Verification items for the finished model (mm, model axes). Coordinates: 2 decimals unless noted, no trailing zeros. Order: outer loops, then holes, each group sorted by start corner. A loop starts at its lowest first (then second) coordinate and runs counter-clockwise, first axis right, second up. Notation, with made-up numbers: (24, 35.25) - (31, 35.25) arc R6 ccw to (31, 41.25) - close; hole circle Ø10 at (60.25, 14). An arc over 180 degrees is marked (long way). One line per question, with ' | ' between items. Start each with the question number.
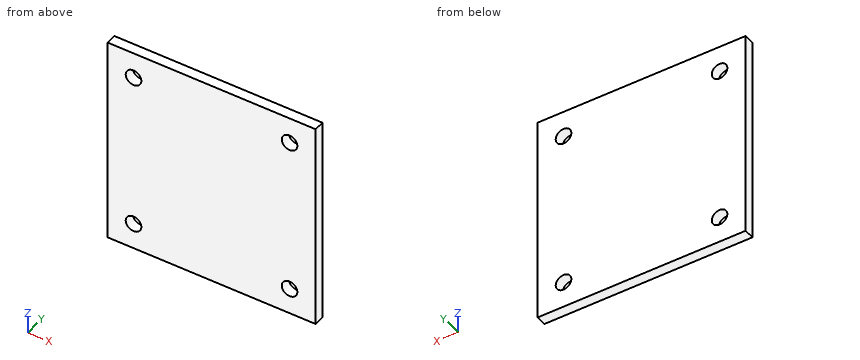
from build123d import *

# Parameters (mm, degrees)
SKETCH1_W           = 40
SKETCH1_H           = 40
BOSS_EXTRUDE1_DEPTH = 2
SKETCH2_R           = 1.5
CUT_EXTRUDE1_DEPTH  = 2


with BuildPart() as part:
    # Sketch1 → Boss-Extrude1 (new body)
    with BuildSketch(Plane(origin=(0, 0, 0), x_dir=(1, 0, 0), z_dir=(0, 1, 0))):
        with Locations((20, 20)):
            Rectangle(SKETCH1_W, SKETCH1_H)
    extrude(amount=BOSS_EXTRUDE1_DEPTH)

    # Sketch2 → Cut-Extrude1 (cut)
    with BuildSketch(Plane.XZ):
        with Locations((35, -5)):
            Circle(SKETCH2_R)
        with Locations((35, -35)):
            Circle(SKETCH2_R)
        with Locations((5, -5)):
            Circle(SKETCH2_R)
        with Locations((5, -35)):
            Circle(SKETCH2_R)
    extrude(amount=-CUT_EXTRUDE1_DEPTH, mode=Mode.SUBTRACT)


solid = part.part
Item 1: Section check C-C (x = 35). Record the cut outline in (y, z), then the cut area to 3 significant figures.
Item 2: Gauge pin test, flat end, axial feed: pin 1 (2.5 mm diameter, centred on x = 5, z = -35, fed in from -Y). Record the tip position at first contact, or that the pin passes through.
Item 3: Section check B-B (z = -5). Record the cut outline in (x, y), then the cut area to 3 significant figures.
Item 4: Section check A-A (y = 1.05). Record the cut outline in (x, z).
Item 5: Thickness scan on probe 1 along Z at (x, y) = (35, 0.6); probe 2 along Z at (x, y) = (4, 1.65); probe 3 along X at (y, z) = (0.35, -4.5). Record the ranges inside material, lowest first. Write a range as from..to.
Completed:
1) outline: (0, -40) - (2, -40) - (2, -36.5) - (0, -36.5) - close; (0, -33.5) - (2, -33.5) - (2, -6.5) - (0, -6.5) - close; (0, -3.5) - (2, -3.5) - (2, 0) - (0, 0) - close | area: 68.0 mm^2
2) pin 1: passes through
3) outline: (0, 0) - (3.5, 0) - (3.5, 2) - (0, 2) - close; (6.5, 0) - (33.5, 0) - (33.5, 2) - (6.5, 2) - close; (36.5, 0) - (40, 0) - (40, 2) - (36.5, 2) - close | area: 68.0 mm^2
4) outline: (0, -40) - (40, -40) - (40, 0) - (0, 0) - close; hole circle Ø3 at (5, -35); hole circle Ø3 at (5, -5); hole circle Ø3 at (35, -35); hole circle Ø3 at (35, -5)
5) probe 1: z = -40..-36.5, -33.5..-6.5, -3.5..0 | probe 2: z = -40..-36.12, -33.88..-6.12, -3.88..0 | probe 3: x = 0..3.59, 6.41..33.59, 36.41..40
